from build123d import *

# Parameters (mm, degrees)
T_LE_DE_BASE_PLI_E1_DEPTH = 100
ESQUISSE6_R               = 2
ENL_V_MAT_EXTRU_1_DEPTH   = 163.225152181


# Read off the part's stored shape, not the designer's step: Tôle de base pliée1
with BuildPart() as part:
    # Tôle de base pliée1 outline → Tôle de base pliée1 (new body)
    with BuildSketch(Plane.XY):
        with BuildLine():
            Line((-126, 0), (-126, -20))
            Line((-126, -20), (-125, -20))
            Line((-125, -20), (-125, 0))
            Line((-125, 0), (125, 0))
            Line((125, 0), (125, -20))
            Line((125, -20), (126, -20))
            Line((126, -20), (126, 0))
            ThreePointArc((126, 0), (125.707106781, 0.707106781), (125, 1))
            Line((125, 1), (-125, 1))
            ThreePointArc((-125, 1), (-125.707106781, 0.707106781), (-126, 0))
        make_face()
    extrude(amount=T_LE_DE_BASE_PLI_E1_DEPTH)

    # Esquisse6 → Enlèv. mat.-Extru.1 (cut, through all)
    with BuildSketch(Plane(origin=(0, 1, 0), x_dir=(1, 0, 0), z_dir=(0, 1, 0))):
        with Locations(Location((0, -10, 0), (0, 0, 180))):
            Circle(ESQUISSE6_R)
    extrude(amount=-ENL_V_MAT_EXTRU_1_DEPTH, mode=Mode.SUBTRACT)


solid = part.part
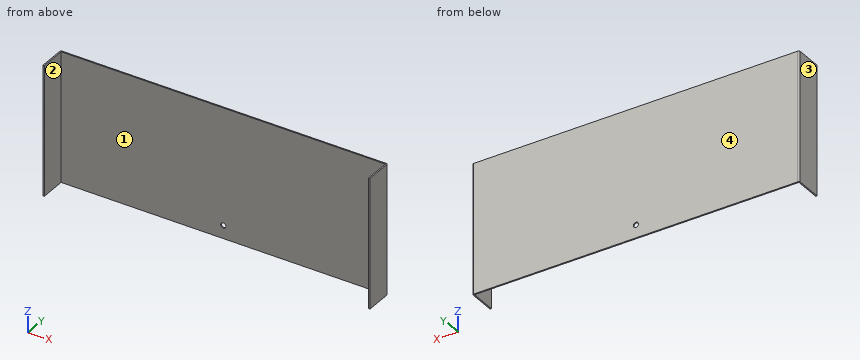
Input: part model. Units: mm. Frame: model coordinates. Face numbers are marked on the shaded views. Round coordinates to 2 decimals unless told otherwise and drop trailing zeros. Order: outer loops, then holes, each group sorted by start corner. A loop starts at its lowest first (then second) coordinate and runs counter-clockwise, first axis right, second up. Notation, with made-up numbers: (47.5, 47.5) - (97.5, 47.5) arc R20 ccw to (97.5, 71.5) - close; hole circle Ø1 at (57.5, 7.25). An arc over 180 degrees is marked (long way). Use a Markdown table: item, result.
1. Section A-A on y = -10.75. Return the cut outline in (x, z).
Evaluation:
| item | result |
|---|---|
| outline | (-126, 0) - (-125, 0) - (-125, 100) - (-126, 100) - close; (125, 0) - (126, 0) - (126, 100) - (125, 100) - close |
2. Material intervals for probe 1 along X at (y, z) = (-17.5, 51); probe 2 along Z at (x, y) = (0, 0.2); probe 3 along Y at (x, z) = (-22, 65.5), sorted ascending.
Evaluation:
| item | result |
|---|---|
| probe 1 | -126 to -125, 125 to 126 |
| probe 2 | 0 to 8, 12 to 100 |
| probe 3 | 0 to 1 |
3. Section B-B on z = 94. Return the cut outline in (x, y), then the cut area to 3 significant figures.
Evaluation:
| item | result |
|---|---|
| outline | (-126, -20) - (-125, -20) - (-125, 0) - (125, 0) - (125, -20) - (126, -20) - (126, 0) arc R1 ccw to (125, 1) - (-125, 1) arc R1 ccw to (-126, 0) - close |
| area | 292 mm^2 |
4. First-contact query: pin 1 (8 mm diameter, centred on x = -24.5, z = 88.5, fed in from -Y). Flat tip, straight axial feed; report the tip coordinate or a pass-through.
Evaluation:
| item | result |
|---|---|
| pin 1 | y = 0 |
5. Section C-C on x = 43. Return the cut outline in (y, z), then the cut area to 3 significant figures.
Evaluation:
| item | result |
|---|---|
| outline | (0, 0) - (1, 0) - (1, 100) - (0, 100) - close |
| area | 100 mm^2 |
6. Mould query, pull axis X, two halves, no side actions, for the marked faces 1, 2, 3 and 4. Classes: +X half, -X half, draft (parallel to the pull), parting line (faces both ways), or undercut.
Evaluation:
| item | result |
|---|---|
| face 1 | undercut |
| face 2 | undercut |
| face 3 | -X half |
| face 4 | draft |
